from build123d import *

# Parameters (mm, degrees)
SKETCH1_R           = 16.8
BOSS_EXTRUDE1_DEPTH = 18.2
SKETCH2_R           = 4
CUT_EXTRUDE1_DEPTH  = 30.928581657
SKETCH3_R           = 1.5
CUT_EXTRUDE2_DEPTH  = 5
SKETCH4_R           = 1.5
CUT_EXTRUDE3_DEPTH  = 5


with BuildPart() as part:
    # Sketch1 → Boss-Extrude1 (new body)
    with BuildSketch(Plane(origin=(0, 0, 0), x_dir=(1, 0, 0), z_dir=(0, 1, 0))):
        with Locations(Location((0, 0, 0), (0, 0, 270))):
            Circle(SKETCH1_R)
    extrude(amount=BOSS_EXTRUDE1_DEPTH)

    # Sketch2 → Cut-Extrude1 (cut, through all)
    with BuildSketch(Plane(origin=(0, 18.2, 0), x_dir=(1, 0, 0), z_dir=(0, 1, 0))):
        with Locations(Location((0, 0, 0), (0, 0, 270))):
            Circle(SKETCH2_R)
    extrude(amount=-CUT_EXTRUDE1_DEPTH, mode=Mode.SUBTRACT)

    # Sketch3 → Cut-Extrude2 (cut)
    with BuildSketch(Plane(origin=(0, 18.2, 0), x_dir=(1, 0, 0), z_dir=(0, 1, 0))):
        with Locations(Location((0, 8, 0), (0, 0, 270))):
            Circle(SKETCH3_R)
        with Locations(Location((8, 0, 0), (0, 0, 270))):
            Circle(SKETCH3_R)
        with Locations(Location((0, -8, 0), (0, 0, 270))):
            Circle(SKETCH3_R)
        with Locations(Location((-8, 0, 0), (0, 0, 270))):
            Circle(SKETCH3_R)
    extrude(amount=-CUT_EXTRUDE2_DEPTH, mode=Mode.SUBTRACT)

    # Sketch4 → Cut-Extrude3 (cut)
    with BuildSketch(Plane.XZ):
        with Locations(Location((0, 11.25, 0), (0, 0, 270))):
            Circle(SKETCH4_R)
        with Locations(Location((11.25, 0, 0), (0, 0, 270))):
            Circle(SKETCH4_R)
        with Locations(Location((0, -11.25, 0), (0, 0, 270))):
            Circle(SKETCH4_R)
        with Locations(Location((-11.25, 0, 0), (0, 0, 270))):
            Circle(SKETCH4_R)
    extrude(amount=-CUT_EXTRUDE3_DEPTH, mode=Mode.SUBTRACT)


solid = part.part
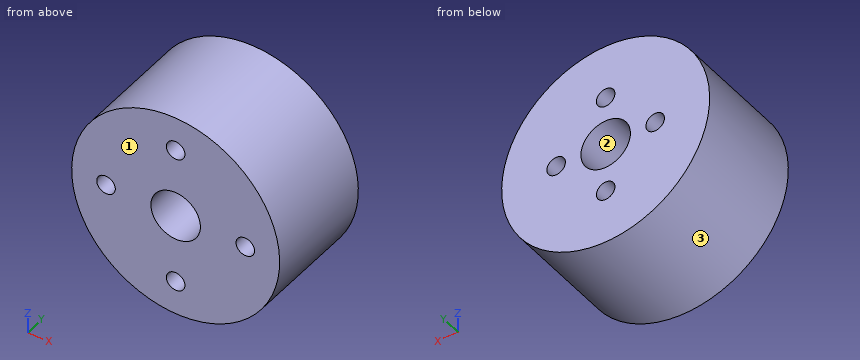
The listing builds one solid part. Answer for the finished solid, in the listing's coordinates (mm). Face numbers are marked on the shaded views. Coordinates: 2 decimals unless noted, no trailing zeros. Loops run counter-clockwise (first coordinate to the right, second up) from the corner with the lowest first, then second, coordinate; pieces in that order, holes last. Notation, with made-up numbers: M 21.5,-16 L 72.5,-16 A23 ccw 72.5,-8 Z; hole C 54,-10 d7. An arc over 180 degrees is marked long. Answer in a Markdown table with one row per item.
1) Given pin 1 (0.9 mm diameter, centred on x = -7.5, z = -0.5, fed in from +Y); pin 2 (10 mm diameter, centred on x = -11, y = 7, fed in from -Z); pin 3 (1.5 mm diameter, centred on x = 11.5, z = 0.5, fed in from -Y), each flat-ended and moving along its own axis, determine where each tip first touches the part or whether it passes through.
Answers below:
| item | result |
|---|---|
| pin 1 | y = 13.2 |
| pin 2 | z = -15.69 |
| pin 3 | y = 5 |
2) Find the intervals of material crossed by probe 1 along Z at (x, y) = (-7.5, 17.25); probe 2 along X at (y, z) = (10, -3.5); probe 3 along Y at (x, z) = (-1, -9), in increasing order.
Answers below:
| item | result |
|---|---|
| probe 1 | -15.03 to -1.41, 1.41 to 15.03 |
| probe 2 | -16.43 to -1.94, 1.94 to 16.43 |
| probe 3 | 0 to 13.2 |
3) Find section C-C (x = 12). Determine the outline of the cut face in (y, z), then the cut area to 3 significant figures.
Answers below:
| item | result |
|---|---|
| outline | M 0,-11.76 L 18.2,-11.76 L 18.2,11.76 L 0,11.76 L 0,1.3 L 5,1.3 L 5,-1.3 L 0,-1.3 Z |
| area | 415 mm^2 |
4) Determine the mould class of the marked faces 1, 2 and 3 for opening direction Z: released by +Z, released by -Z, zero draft, split by the parting line, or undercut.
Answers below:
| item | result |
|---|---|
| face 1 | zero draft |
| face 2 | undercut |
| face 3 | split by the parting line |
5) Find section B-B (y = 3). Determine the outline of the cut face in (x, z).
Answers below:
| item | result |
|---|---|
| outline | C 0,0 d33.6; hole C -11.25,0 d3; hole C 0,0 d8; hole C 0,-11.25 d3; hole C 0,11.25 d3; hole C 11.25,0 d3 |
6) Find section A-A (z = 0). Determine the outline of the cut face in (x, y), then the cut area to 3 significant figures.
Answers below:
| item | result |
|---|---|
| outline | M -16.8,0 L -12.75,0 L -12.75,5 L -9.75,5 L -9.75,0 L -4,0 L -4,18.2 L -6.5,18.2 L -6.5,13.2 L -9.5,13.2 L -9.5,18.2 L -16.8,18.2 Z; M 4,0 L 9.75,0 L 9.75,5 L 12.75,5 L 12.75,0 L 16.8,0 L 16.8,18.2 L 9.5,18.2 L 9.5,13.2 L 6.5,13.2 L 6.5,18.2 L 4,18.2 Z |
| area | 406 mm^2 |
7) Find section D-D (z = -7). Determine the outline of the cut face in (x, y), then the cut area to 3 significant figures.
Answers below:
| item | result |
|---|---|
| outline | M -15.27,0 L 15.27,0 L 15.27,18.2 L 1.12,18.2 L 1.12,13.2 L -1.12,13.2 L -1.12,18.2 L -15.27,18.2 Z |
| area | 545 mm^2 |
